Build history of the part. All positions in model axes, mm. Face numbers are marked on the shaded views. Round coordinates to 2 decimals unless told otherwise and drop trailing zeros. Write each loop counter-clockwise with the first axis right and the second up, starting at its lowest first coordinate (ties: lowest second). Pieces come first, ordered by that corner, then holes. Notation, with made-up numbers: (41.25, 4) -> (54.25, 4) arc R16 ccw to (54.25, 9) -> close; hole circle Ø5 at (-9, 25). An arc over 180 degrees is marked (long way). Answer as CSV lines item,"result".
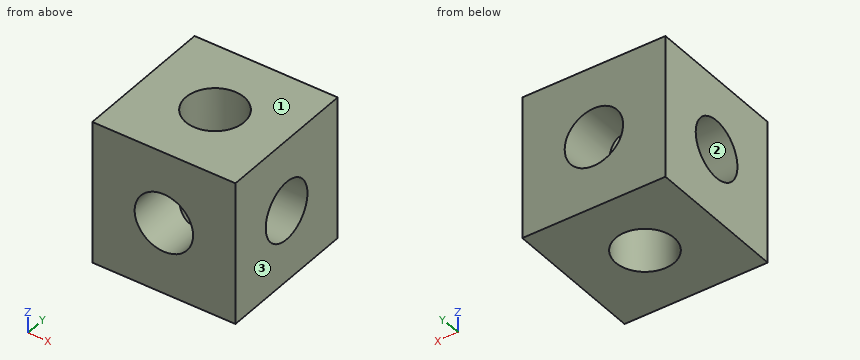
from build123d import *

# Parameters (mm, degrees)
F0_W          = 24.5
F0_H          = 24.5
F0_R          = 5
F1_DEPTH      = 12.25
F2_R          = 5
F3_DEPTH      = 12.251
F3_DEPTH_BACK = 12.251
F4_R          = 5
F5_DEPTH      = 12.251
F5_DEPTH_BACK = 12.251


with BuildPart() as f1:
    # F0 (on Front) → F1 (new body, symmetric)
    with BuildSketch(Plane.XZ):
        Rectangle(F0_W, F0_H)
        Circle(F0_R, mode=Mode.SUBTRACT)
    extrude(amount=F1_DEPTH, both=True)

    # F2 (on Right) → F3 (cut, two sides)
    with BuildSketch(Plane.YZ) as f3_sk:
        Circle(F2_R)
    extrude(amount=-F3_DEPTH, mode=Mode.SUBTRACT)
    extrude(f3_sk.sketch, amount=F3_DEPTH_BACK, mode=Mode.SUBTRACT)

    # F4 (on Top) → F5 (cut, two sides)
    with BuildSketch(Plane.XY) as f5_sk:
        Circle(F4_R)
    extrude(amount=-F5_DEPTH, mode=Mode.SUBTRACT)
    extrude(f5_sk.sketch, amount=F5_DEPTH_BACK, mode=Mode.SUBTRACT)


solid = f1.part
1. Cut at C-C, the plane z = 4.25. Write the cut outline in (x, y).
Results found:
outline,"(-12.25, -12.25) -> (-2.63, -12.25) -> (-2.63, -4.25) arc R5 cw to (-4.25, -2.63) -> (-12.25, -2.63) -> close; (-12.25, 2.63) -> (-4.25, 2.63) arc R5 cw to (-2.63, 4.25) -> (-2.63, 12.25) -> (-12.25, 12.25) -> close; (2.63, -12.25) -> (12.25, -12.25) -> (12.25, -2.63) -> (4.25, -2.63) arc R5 cw to (2.63, -4.25) -> close; (2.63, 4.25) arc R5 cw to (4.25, 2.63) -> (12.25, 2.63) -> (12.25, 12.25) -> (2.63, 12.25) -> close"
2. Probe line 1 along X through (y, z) = (9.75, 0); line 2 along X through (y, z) = (-8.5, 4.5). List the from-to ranges inside material, lowest first.
Results found:
line 1,"x = -12.25 to -5, 5 to 12.25"
line 2,"x = -12.25 to -2.18, 2.18 to 12.25"
3. Cut at D-D, the plane x = -9.75. Write the cut outline in (y, z), then the cut area to 3 significant figures.
Results found:
outline,"(-12.25, -12.25) -> (12.25, -12.25) -> (12.25, 12.25) -> (-12.25, 12.25) -> close; hole circle Ø10 at (0, 0)"
area,"522 mm2"
4. Cut at A-A, the plane y = 0. Write the cut outline in (x, z).
Results found:
outline,"(-12.25, -12.25) -> (-5, -12.25) -> (-5, -5) -> (-12.25, -5) -> close; (-12.25, 5) -> (-5, 5) -> (-5, 12.25) -> (-12.25, 12.25) -> close; (5, -12.25) -> (12.25, -12.25) -> (12.25, -5) -> (5, -5) -> close; (5, 5) -> (12.25, 5) -> (12.25, 12.25) -> (5, 12.25) -> close"
5. Mould opens along Z. For the marked faces 1, 2 and 3 say: +Z half, -Z half, draft (parallel to the pull), parting line (faces both ways), or undercut.
Results found:
face 1,"+Z half"
face 2,"undercut"
face 3,"draft"
